```python
from build123d import *

# Parameters (mm, degrees)
SKETCH1_W                  = 60
SKETCH1_H                  = 60
BOSS_EXTRUDE1_DEPTH        = 3
F_2_5_2_5_DIAMETER_HOLE1_D = 2.5


with BuildPart() as part:
    # Sketch1 → Boss-Extrude1 (new body)
    with BuildSketch(Plane(origin=(0, 0, -7), x_dir=(-1, 0, 0), z_dir=(0, 0, -1))):
        Rectangle(SKETCH1_W, SKETCH1_H)
    extrude(amount=-BOSS_EXTRUDE1_DEPTH)

    # Ø2.5 (2.5) Diameter Hole1 (through all)
    with Locations(Plane.XY.offset(-4)):
        with Locations((-27, 27), (-27, -27), (27, -27), (27, 27)):
            Hole(F_2_5_2_5_DIAMETER_HOLE1_D / 2)


solid = part.part
```
Check sheet for the modelled part. Datum: model origin and axes. Units: mm. Give positions to 0.01 mm unless a question says otherwise; leave off trailing zeros. Loops run counter-clockwise (first coordinate to the right, second up) from the corner with the lowest first, then second, coordinate; pieces in that order, holes last. Notation, with made-up numbers: M 84,44.5 L 101,44.5 A29 cw 101,83.5 Z; hole C 69.25,41.5 d11. An arc over 180 degrees is marked long. Answer in a Markdown table with one row per item.
1) Depth check by flat-ended pin: pin 1 (3 mm diameter, centred on x = -27, y = 27, fed in from +Z). Enter the tip coordinate at first touch or a pass-through.
Solutions:
| item | result |
|---|---|
| pin 1 | stops at z = -4 |
2) Cross-section at A-A (x = -27). Enter the section's corners in (y, z), plus the area to 3 significant figures.
Solutions:
| item | result |
|---|---|
| outline | M -30,-7 L -28.25,-7 L -28.25,-4 L -30,-4 Z; M -25.75,-7 L 25.75,-7 L 25.75,-4 L -25.75,-4 Z; M 28.25,-7 L 30,-7 L 30,-4 L 28.25,-4 Z |
| area | 165 mm^2 |
3) Thickness scan on line 1 (Y direction, x = 27, z = -6.15); line 2 (X direction, y = 26, z = -4.6); line 3 (Y direction, x = 27.5, z = -4.95). Record the ranges inside material, lowest first.
Solutions:
| item | result |
|---|---|
| line 1 | y = -30 to -28.25, -25.75 to 25.75, 28.25 to 30 |
| line 2 | x = -30 to -27.75, -26.25 to 26.25, 27.75 to 30 |
| line 3 | y = -30 to -28.15, -25.85 to 25.85, 28.15 to 30 |
4) Mould release check, pull along X, two halves, no side actions. Record for faces 1 (the face through (0, 30, -6)), 2 (the face through (25.845, -27.479, -5.521)), 3 (the face through (-30, 0, -6)): released by +X, released by -X, zero draft, split by the parting line, or undercut.
Solutions:
| item | result |
|---|---|
| face 1 | zero draft |
| face 2 | undercut |
| face 3 | released by -X |
